Geometry check sheet. Reference: the model listing, model coordinates, mm. Face numbers are marked on the shaded views. A direction names the side the tool comes from. Give positions to 0.01 mm unless a question says otherwise; leave off trailing zeros. Loops run counter-clockwise (first coordinate to the right, second up) from the corner with the lowest first, then second, coordinate; pieces in that order, holes last. Notation, with made-up numbers: (36.5, -28.75) -> (81.5, -28.75) arc R21 ccw to (81.5, -6.75) -> close; hole circle Ø8 at (77, -12). An arc over 180 degrees is marked (long way). Answer in a Markdown table with one row per item. Add a question column.
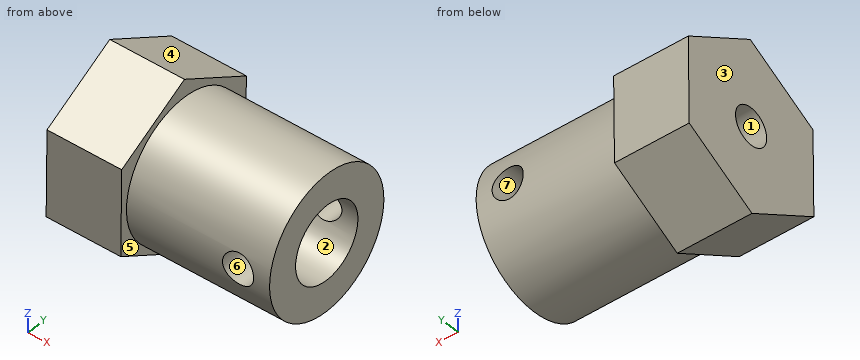
```python
from build123d import *

# Parameters (mm, degrees)
SKETCH1_R           = 5.5
BOSS_EXTRUDE1_DEPTH = 11.5
BOSS_EXTRUDE2_DEPTH = 6
SKETCH3_R           = 3
CUT_EXTRUDE1_DEPTH  = 10
SKETCH4_R           = 1.25
CUT_EXTRUDE4_DEPTH  = 10
SKETCH5_R           = 1.5
CUT_EXTRUDE5_DEPTH  = 5


with BuildPart() as part:
    # Sketch1 → Boss-Extrude1 (new body)
    with BuildSketch(Plane(origin=(0, 0, 0), x_dir=(0, 0, -1), z_dir=(1, 0, 0))):
        Circle(SKETCH1_R)
    extrude(amount=BOSS_EXTRUDE1_DEPTH)

    # Sketch2 → Boss-Extrude2 (add)
    with BuildSketch(Plane.ZY):
        Polygon((3.392309556, 6.040880389), (-3.535401101, 5.958266447), (-6.927710656, -0.082613942), (-3.392309556, -6.040880389), (3.535401101, -5.958266447), (6.927710656, 0.082613942), align=None)
    extrude(amount=BOSS_EXTRUDE2_DEPTH)

    # Sketch3 → Cut-Extrude1 (cut)
    with BuildSketch(Plane(origin=(11.5, 0, 0), x_dir=(0, 0, -1), z_dir=(1, 0, 0))):
        Circle(SKETCH3_R)
    extrude(amount=-CUT_EXTRUDE1_DEPTH, mode=Mode.SUBTRACT)

    # Sketch4 → Cut-Extrude4 (cut, symmetric)
    with BuildSketch(Plane(origin=(0, 0, 0), x_dir=(1, 0, 0), z_dir=(0, 1, 0))):
        with Locations(Location((8.965402785, 0, 0), (0, 0, 270))):
            Circle(SKETCH4_R)
    extrude(amount=CUT_EXTRUDE4_DEPTH, both=True, mode=Mode.SUBTRACT)

    # Sketch5 → Cut-Extrude5 (cut)
    with BuildSketch(Plane.ZY.offset(6)):
        Circle(SKETCH5_R)
    extrude(amount=-CUT_EXTRUDE5_DEPTH, mode=Mode.SUBTRACT)


solid = part.part
```
1. Sectioned sample at C-C (x = -0.25). Enter the section's corners in (y, z).
2. Release check for a two-part mould opening along Z. For the marked faces 4, 5, 6 and 7 record: released by +Z, released by -Z, zero draft, split by the parting line, or undercut.
3. Sectioned sample at A-A (z = 0). Enter the section's corners in (x, y), plus the area to 3 significant figures.
4. Gauge pin test, flat ends, axial feed: pin 1 Ø3.5 at (y, z) = (0, 0) entering from +X; pin 2 Ø1.5 at (x, y) = (0, -3) entering from +Z; pin 3 Ø1.5 at (x, z) = (8.97, 0) entering from -Y; pin 4 Ø1 at (x, z) = (5, -1) entering from +Y. Record the tip position at first contact, or that the pin passes through.
5. Material ranges on L1, parallel to X at y = -4.2, z = 0; L2, parallel to Z at x = 2.25, y = 1.5; L3, parallel to X at y = 0.75, z = 0, recorded low to high. Write a range as from..to.
6. Sectioned sample at D-D (x = 2.75). Enter the section's corners in (y, z).
7. Sectioned sample at B-B (y = 4). Enter the section's corners in (x, z), plus the area to 3 significant figures.
8. Access from +Z, -Z, +X, -X, +Y, -Y to the whole of each face (thin tool, end or side, straight path). Record for the marked faces 1, 2 and 3.
Response:
| question | item | result |
|---|---|---|
| 1 | outline | (-6.04, -3.39) -> (-0.08, -6.93) -> (5.96, -3.54) -> (6.04, 3.39) -> (0.08, 6.93) -> (-5.96, 3.54) -> close |
| 2 | face 4 | released by +Z |
| 2 | face 5 | zero draft |
| 2 | face 6 | undercut |
| 2 | face 7 | undercut |
| 3 | outline | (-6, -6) -> (0, -6) -> (0, -5.5) -> (7.72, -5.5) -> (7.72, -3) -> (1.5, -3) -> (1.5, 3) -> (7.72, 3) -> (7.72, 5.5) -> (0, 5.5) -> (0, 6) -> (-6, 6) -> (-6, 1.5) -> (-1, 1.5) -> (-1, -1.5) -> (-6, -1.5) -> close; (10.22, -5.5) -> (11.5, -5.5) -> (11.5, -3) -> (10.22, -3) -> close; (10.22, 3) -> (11.5, 3) -> (11.5, 5.5) -> (10.22, 5.5) -> close |
| 3 | area | 111 mm2 |
| 4 | pin 1 | stops at x = 1.5 |
| 4 | pin 2 | stops at z = 5.62 |
| 4 | pin 3 | passes through |
| 4 | pin 4 | stops at y = 5.48 |
| 5 | L1 | x = -6..7.72, 10.22..11.5 |
| 5 | L2 | z = -5.29..-2.6, 2.6..5.29 |
| 5 | L3 | x = -1..1.5 |
| 6 | outline | circle Ø11 at (0, 0); hole circle Ø6 at (0, 0) |
| 7 | outline | (-6, -4.64) -> (0, -4.64) -> (0, -3.77) -> (11.5, -3.77) -> (11.5, 3.77) -> (0, 3.77) -> (0, 4.6) -> (-6, 4.6) -> close; hole circle Ø2.5 at (8.97, 0) |
| 7 | area | 137 mm2 |
| 8 | face 1 | -X |
| 8 | face 2 | +X |
| 8 | face 3 | +Z, -Z, -X, +Y, -Y |
